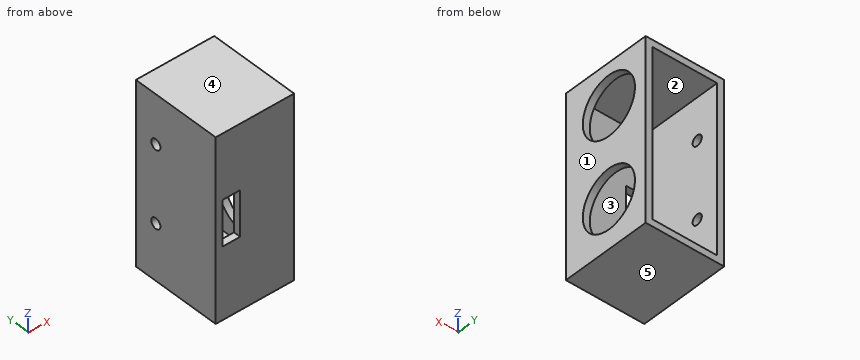
Autodesk Inventor part; units mm, degrees
ref_plane "YZ Plane" through (0, 0, 0) normal (1, 0, 0) x (0, 1, 0)
ref_plane "XZ Plane" through (0, 0, 0) normal (0, 1, 0) x (-1, 0, 0)
ref_plane "XY Plane" through (0, 0, 0) normal (0, 0, 1) x (1, 0, 0)
sketch "Sketch1" plane through (0, 0, 0) normal (1, 0, 0) x (0, 1, 0)
  line L0 (0, 0) -> (0, -52)
  line L1 (0, -52) -> (26, -52)
  line L2 (26, -52) -> (26, 0)
  line L3 (26, 0) -> (0, 0)
  line L4 (26, 0) -> (19.5, 0)
  line L5 (19.5, 0) -> (19.5, -14)
  line L6 (19.5, -14) -> (19.5, -36)
  circle A0 centre (19.5, -14) radius 1.5
  circle A1 centre (19.5, -36) radius 1.5
  dimension "d0" = 52
  dimension "d1" = 26
  dimension "d2" = 6.5
  dimension "d3" = 14
  dimension "d4" = 22
  dimension "d5" = 3
  dimension "d6" = 3
extrude "Extrusion1" add sketch "Sketch1" along normal blind 2
sketch "Sketch2" plane through (2, 0, 0) normal (1, 0, 0) x (0, 0, -1)
  line L0 (0, 0) -> (52, 0)
  line L1 (52, 0) -> (52, 26)
  line L2 (52, 26) -> (0, 26)
  line L3 (0, 26) -> (0, 0)
  circle A0 centre (36, 19.5) radius 1.5
  circle A1 centre (14, 19.5) radius 1.5
  line L4 (52, 26) -> (0, 26)
  line L5 (0, 26) -> (2, 26)
  line L6 (2, 26) -> (2, 2)
  line L7 (2, 2) -> (50, 2)
  line L8 (50, 2) -> (50, 24)
  line L9 (50, 24) -> (2, 24)
  line L10 (50, 24) -> (50, 26)
  dimension "d9" = 2
  dimension "d10" = 24
  dimension "d11" = 48
  dimension "d12" = 22
extrude "Extrusion2" add sketch "Sketch2" along normal blind 17 contours L3 L2 L6 L7 L8 L10 L1 L0
sketch "Sketch3" plane through (19, 0, 0) normal (1, 0, 0) x (0, 0, -1)
  line L0 (52, 26) -> (50, 26)
  line L1 (50, 26) -> (50, 2)
  line L2 (50, 2) -> (2, 2)
  line L3 (2, 2) -> (2, 26)
  line L4 (2, 26) -> (0, 26)
  line L5 (0, 26) -> (0, 0)
  line L6 (0, 0) -> (52, 0)
  line L7 (52, 0) -> (52, 26)
  line L8 (2, 26) -> (0, 26)
  line L9 (52, 26) -> (0, 26)
  line L10 (0, 26) -> (52, 26)
extrude "Extrusion3" add sketch "Sketch3" along normal blind 2
sketch "Sketch4" plane through (21, 0, 0) normal (1, 0, 0) x (0, 0, -1)
  circle A0 centre (14, 19.5) radius 1.5
  line L0 (52, 26) -> (0, 26)
  line L1 (0, 26) -> (0, 0)
  line L2 (0, 0) -> (52, 0)
  line L3 (52, 0) -> (52, 26)
  circle A1 centre (36, 19.5) radius 1.5
  line L4 (52, 26) -> (0, 26)
  line L5 (0, 26) -> (0, 0)
  line L6 (0, 0) -> (52, 0)
  line L7 (52, 0) -> (52, 26)
  line L8 (0, 26) -> (0, 0)
  line L9 (0, 26) -> (25, 26)
  line L10 (50, 26) -> (2, 26)
  line L11 (25, 26) -> (38, 26)
  line L12 (38, 26) -> (38, 0)
  line L13 (0, 0) -> (52, 0)
  line L14 (25, 26) -> (12, 26)
  line L15 (12, 26) -> (12, 0)
  line L16 (52, 26) -> (0, 26)
  line L17 (0, 26) -> (0, 4)
  line L18 (0, 4) -> (50, 4)
  line L19 (52, 0) -> (52, 26)
  line L20 (50, 4) -> (50, 26)
  line L21 (0, 26) -> (0, 24)
  line L22 (0, 24) -> (0, 14)
  line L23 (0, 14) -> (38, 14)
  circle A2 centre (12, 14) radius 8.5
  circle A3 centre (38, 14) radius 8.5
  dimension "d17" = 25
  dimension "d18" = 13
  dimension "d19" = 13
  dimension "d20" = 22
  dimension "d21" = 2
  dimension "d22" = 10
  dimension "d23" = 17
  dimension "d24" = 17
extrude "Extrusion4" cut sketch "Sketch4" against normal blind 2 contours A0 | A3 L12 | L12 L23 A3 | L12 A3 L23 | A2 L23 L15 | L15 L23 A2 | A2 L15 L23 | A2 L23 L15 | A1
sketch "Sketch5" plane through (2, 2, -2) normal (0, 1, 0) x (1, 0, 0)
  line L0 (0, 0) -> (0, 48)
  line L1 (0, 0) -> (17, 0)
  line L2 (17, 48) -> (17, 0)
  line L3 (0, 48) -> (17, 48)
  line L4 (0, 13.5) -> (0, 10.5)
  line L5 (0, 35.5) -> (0, 32.5)
  line L6 (0, 48) -> (0, 0)
  line L7 (0, 0) -> (0, 12)
  line L8 (0, 12) -> (0, 34)
  line L9 (0, 12) -> (0, 23)
  line L10 (0, 23) -> (0, 29.5)
  line L11 (0, 29.5) -> (4, 29.5)
  line L12 (4, 29.5) -> (4, 16.5)
  line L13 (4, 16.5) -> (0, 16.5)
  line L14 (0, 16.5) -> (0, 23)
  point P0 (-2, -2)
  point P1 (0, 16.5)
  dimension "d27" = 12
  dimension "d28" = 22
  dimension "d29" = 11
  dimension "d30" = 6.5
  dimension "d31" = 4
  dimension "d32" = 13
extrude "Extrusion5" cut sketch "Sketch5" against normal blind 2 contours L0 L11 L12 L13
sketch "Sketch6" plane through (21, 0, 0) normal (1, 0, 0) x (0, 0, -1)
  circle A0 centre (38, 14) radius 8.5
  circle A1 centre (12, 14) radius 8.5
  line L0 (52, 26) -> (0, 26)
  line L1 (0, 26) -> (0, 0)
  line L2 (0, 0) -> (52, 0)
  line L3 (52, 0) -> (52, 26)
extrude "Extrusion6" add sketch "Sketch6" along normal blind 1.5
sketch "Sketch7" plane through (19, 0, 0) normal (-1, 0, 0) x (0, 0, 1)
  line L0 (0, 26) -> (0, 0)
  line L1 (0, 0) -> (-52, 0)
  line L2 (-52, 0) -> (-52, 26)
  line L3 (-52, 26) -> (0, 26)
  circle A0 centre (-38, 14) radius 8.5
  circle A1 centre (-12, 14) radius 8.5
  line L4 (0, 26) -> (0, 0)
  line L5 (0, 26) -> (-2, 26)
  line L6 (-52, 26) -> (0, 26)
  line L7 (-2, 26) -> (-2, 2)
  line L8 (-2, 2) -> (-50, 2)
  line L9 (-50, 2) -> (-50, 26)
  dimension "d37" = 2
  dimension "d38" = 24
  dimension "d39" = 48
extrude "Extrusion7" cut sketch "Sketch7" against normal blind 1.5 contours L7 L8 L9 L3
sketch "Sketch8" plane through (2, 2, -31.5) normal (0, 1, 0) x (1, 0, 0)
  line L0 (0, 0) -> (4, 0)
  line L1 (4, 0) -> (4, -13)
  line L2 (4, -13) -> (0, -13)
  line L3 (0, -29.5) -> (0, -13)
  line L4 (0, -29.5) -> (18.5, -29.5)
  line L5 (18.5, -29.5) -> (18.5, 18.5)
  line L6 (0, 18.5) -> (18.5, 18.5)
  line L7 (0, 0) -> (0, 18.5)
  line L8 (4, -13) -> (0, -13)
  line L9 (4, -13) -> (5, -13)
  line L10 (5, -13) -> (5, 0)
  line L11 (4, 0) -> (4, -13)
  line L12 (5, 0) -> (4, 0)
  point P0 (-2, -31.5)
  dimension "d42" = 1
extrude "Extrusion8" cut sketch "Sketch8" against normal through all contours L12 L10 L9 L1
properties part number "soporte_sensor"
Check sheet for the modelled part. Datum: model origin and axes. Units: mm. Face numbers are marked on the shaded views. A direction names the side the tool comes from. Give positions to 0.01 mm unless a question says otherwise; leave off trailing zeros. Write each loop counter-clockwise with the first axis right and the second up, starting at its lowest first coordinate (ties: lowest second). Pieces come first, ordered by that corner, then holes. Notation, with made-up numbers: (78.5, -1.75) -> (90.5, -1.75) arc R10 ccw to (90.5, 17.25) -> close; hole circle Ø9 at (81.25, 18). An arc over 180 degrees is marked (long way). Use one line per item in the form item = value. Start each with the question number.
1. Section check B-B (y = 10). Record the cut outline in (x, z), and give its area (3 significant figures).
2. Thickness scan on line 1 along Z through (x, y) = (21.45, 14); line 2 along Y through (x, z) = (21.1, -12); line 3 along Y through (x, z) = (1.25, -36). Record the ranges inside material, lowest first. Write a range as from..to.
3. Section check C-C (x = 20). Record the cut outline in (y, z), and give its area (3 significant figures).
4. Go/stop test with flat-tipped pins: P1, Ø1, axis at x = 5, y = 1, coming from the +Z side; P2, Ø1, axis at y = 14.5, z = -17.5, coming from the +X side. Record where each tip stops, or that it passes through.
5. Mould release check, pull along Z, two halves, no side actions. Record for the marked faces 3, 4 and 5: pulls with the +Z half, pulls with the -Z half, needs draft (parallel to the pull), parting line crosses it, or undercut.
6. Section check D-D (y = 24.75). Record the cut outline in (x, z), and give its area (3 significant figures).
7. Section check A-A (z = -42). Record the cut outline in (x, y).
8. Access from +Z, -Z, +X, -X, +Y, -Y to the whole of each face (thin tool, end or side, straight path). Record for the marked faces 1 and 2.
Conclusion:
q1.outline = (0, -52) -> (22.5, -52) -> (22.5, -45.5) -> (20.5, -45.5) -> (20.5, -50) -> (2, -50) -> (2, -2) -> (20.5, -2) -> (20.5, -4.5) -> (22.5, -4.5) -> (22.5, 0) -> (0, 0) -> close; (20.5, -30.5) -> (22.5, -30.5) -> (22.5, -19.5) -> (20.5, -19.5) -> close
q1.area = 222 mm²
q2.line_1 = -52..-46.5, -29.5..-20.5, -3.5..0
q2.line_2 = 0..5.5, 22.5..26
q2.line_3 = 0..18, 21..26
q3.outline = (0, -52) -> (26, -52) -> (26, -50) -> (2, -50) -> (2, -2) -> (26, -2) -> (26, 0) -> (0, 0) -> close
q3.area = 200 mm²
q4.P1 = 0
q4.P2 = 2
q5.face_3 = undercut
q5.face_4 = pulls with the +Z half
q5.face_5 = pulls with the -Z half
q6.outline = (0, -52) -> (22.5, -52) -> (22.5, 0) -> (0, 0) -> close; hole (2, -50) -> (20.5, -50) -> (20.5, -2) -> (2, -2) -> close
q6.area = 282 mm²
q7.outline = (0, 0) -> (22.5, 0) -> (22.5, 6.5) -> (20.5, 6.5) -> (20.5, 2) -> (2, 2) -> (2, 26) -> (0, 26) -> close; (20.5, 21.5) -> (22.5, 21.5) -> (22.5, 26) -> (20.5, 26) -> close
q8.face_1 = +Z, -Z, +X, +Y, -Y
q8.face_2 = +Y
